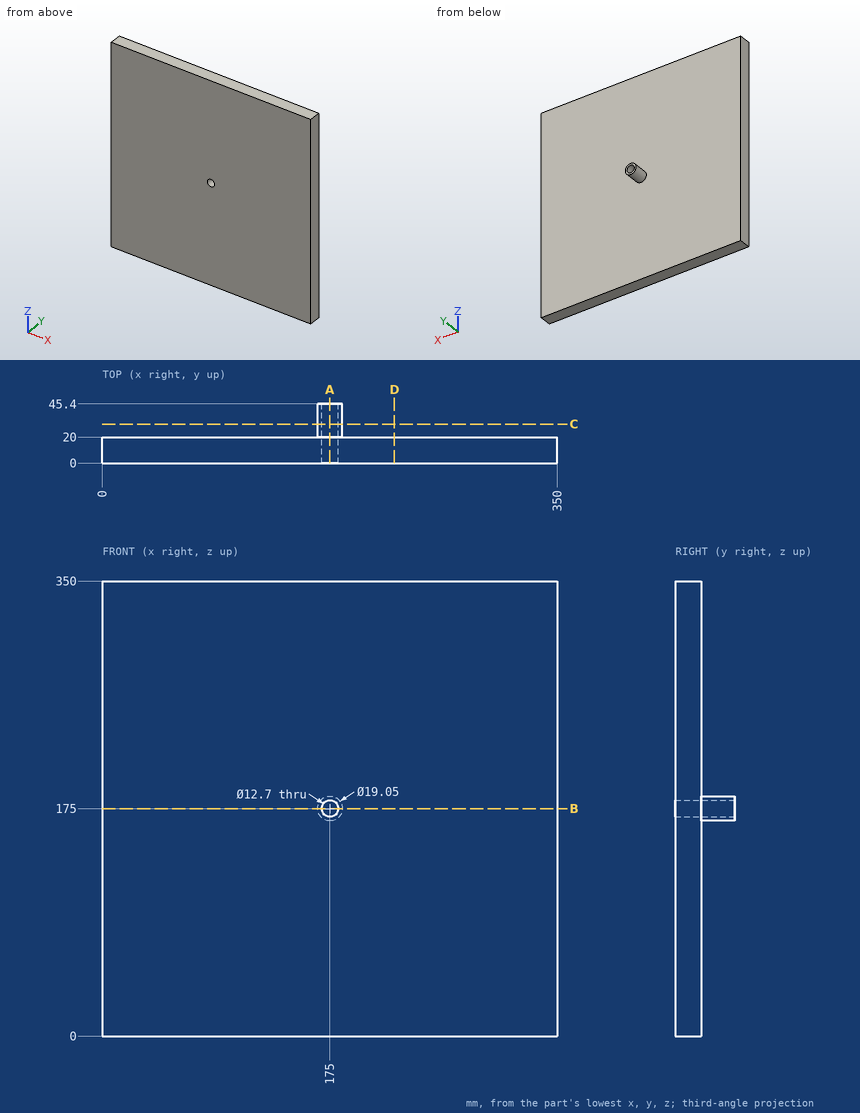
The drawing under review shows one solid part. Ordinate dimensions are in mm from its lowest x, y, z. Round coordinates to 2 decimals unless told otherwise and drop trailing zeros. Write each loop counter-clockwise with the first axis right and the second up, starting at its lowest first coordinate (ties: lowest second). Pieces come first, ordered by that corner, then holes. Notation, with made-up numbers: (-21.5, 88.25) -> (19.5, 88.25) arc R16 cw to (19.5, 109.25) -> close; hole circle Ø6 at (68.25, 87). An arc over 180 degrees is marked (long way). Put each result on its own line as item: value.
Q1. Consider section A-A on x = 175. State the section outline as (y, z) points (3 decimals).
Determined:
outline: (0, 0) -> (20, 0) -> (20, 165.475) -> (45.4, 165.475) -> (45.4, 168.65) -> (0, 168.65) -> close; (0, 181.35) -> (45.4, 181.35) -> (45.4, 184.525) -> (20, 184.525) -> (20, 350) -> (0, 350) -> close
Q2. Consider section B-B on z = 175. State the section outline as (x, y) points (3 decimals), and give its area (3 significant figures).
Determined:
outline: (0, 0) -> (168.65, 0) -> (168.65, 45.4) -> (165.475, 45.4) -> (165.475, 20) -> (0, 20) -> close; (181.35, 0) -> (350, 0) -> (350, 20) -> (184.525, 20) -> (184.525, 45.4) -> (181.35, 45.4) -> close
area: 6,910 mm^2
Q3. Clearance check with a flat-ended pin moving along its axis: pin 1 Ø1 at (x, z) = (133.5, 236) entering from +Y. State where the tip first meets the part, or that it passes through.
Determined:
pin 1: stops at y = 20
Q4. Consider section C-C on y = 30. State the section outline as (x, z) points (3 decimals).
Determined:
outline: circle Ø19.05 at (175, 175); hole circle Ø12.7 at (175, 175)
Q5. To check wall thickness, follow L1, parallel to X at y = 31, z = 175 (3 decimals); L2, parallel to Y at x = 137, z = 108; L3, parallel to X at y = 39.5, z = 183.5. State the ranges of each line that lie inside material, in increasing order. Write a range as [from, to].
Determined:
L1: x = [165.475, 168.65], [181.35, 184.525]
L2: y = [0, 20]
L3: x = [170.7, 179.3]
Q6. Consider section D-D on x = 224.5. State the section outline as (y, z) points.
Determined:
outline: (0, 0) -> (20, 0) -> (20, 350) -> (0, 350) -> close
